Drawing for the job (mm, zero at the part's lowest x, y, z). A direction names the side the tool comes from. Coordinates: 2 decimals unless noted, no trailing zeros. Order: outer loops, then holes, each group sorted by start corner. A loop starts at its lowest first (then second) coordinate and runs counter-clockwise, first axis right, second up. Notation, with made-up numbers: (-12.75, -33.75) -> (16.25, -33.75) arc R11 cw to (16.25, -15.75) -> close; hole circle Ø11 at (35, 43). An arc over 180 degrees is marked (long way). Write each question's results on one line, items separated by ' | '.
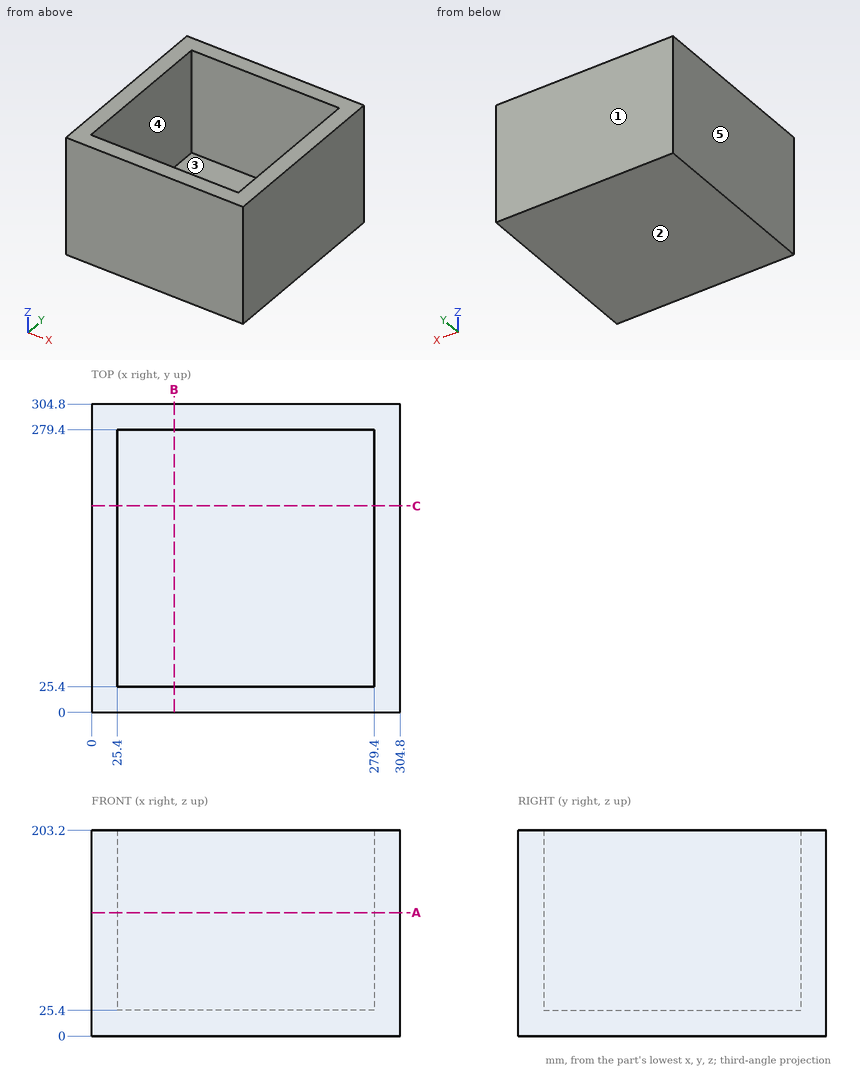
Item 1: Slice it at A-A, the plane z = 122. List the corners of the cut face in (x, y), and give its area (3 significant figures).
Answer:
outline: (0, 0) -> (304.8, 0) -> (304.8, 304.8) -> (0, 304.8) -> close; hole (25.4, 25.4) -> (279.4, 25.4) -> (279.4, 279.4) -> (25.4, 279.4) -> close | area: 28,400 mm^2
Item 2: Drill centre lines: line 1 (Y direction, x = 235, z = 88.5); line 2 (Z direction, x = 237, y = 256.5). Where is each one in solid material? Low to high. Write a range as from..to.
Answer:
line 1: y = 0..25.4, 279.4..304.8 | line 2: z = 0..25.4
Item 3: Pull direction Y, two halves, no side cores. Call the marked faces 1, 2 and 3: released by +Y, released by -Y, zero draft, split by the parting line, or undercut.
Answer:
face 1: released by +Y | face 2: zero draft | face 3: undercut
Item 4: Tool access for the marked faces 4 and 5: list every direction of +Z, -Z, +X, -X, +Y, -Y with a clear straight run to the whole face (end or side of a thin tool).
Answer:
face 4: +Z | face 5: +Z, -Z, -X, +Y, -Y
Item 5: Pin check, flat tip, straight feed: pin 1 (1 mm diameter, centred on x = 110, y = 258.5, fed in from +Z). Stop position of the tip, or through.
Answer:
pin 1: stops at z = 25.4
Item 6: Slice it at B-B, the plane x = 81.5. List the corners of the cut face in (y, z), and give its area (3 significant figures).
Answer:
outline: (0, 0) -> (304.8, 0) -> (304.8, 203.2) -> (279.4, 203.2) -> (279.4, 25.4) -> (25.4, 25.4) -> (25.4, 203.2) -> (0, 203.2) -> close | area: 16,800 mm^2
